from build123d import *

# Parameters (mm, degrees)
SKETCH1_W           = 59.055
SKETCH1_H           = 28.448
BOSS_EXTRUDE1_DEPTH = 46.482
SKETCH2_R           = 2.54
BOSS_EXTRUDE2_DEPTH = 3.81
FILLET1_R           = 2.54
CHAMFER1_SIZE       = 1.778


with BuildPart() as part:
    # Sketch1 → Boss-Extrude1 (new body)
    with BuildSketch(Plane(origin=(0, 0, 0), x_dir=(1, 0, 0), z_dir=(0, 1, 0))):
        with Locations((-2.344011553, -9.758904569)):
            Rectangle(SKETCH1_W, SKETCH1_H)
    extrude(amount=BOSS_EXTRUDE1_DEPTH)

    # Sketch2 → Boss-Extrude2 (add)
    with BuildSketch(Plane(origin=(0, 46.482, 0), x_dir=(1, 0, 0), z_dir=(0, 1, 0))):
        with Locations(Location((14.483488447, -9.758904569, 0), (0, 0, 90))):
            Circle(SKETCH2_R)
    extrude(amount=BOSS_EXTRUDE2_DEPTH)

    # Fillet1
    fillet1_edges = [part.edges().sort_by_distance(p)[0] for p in [
        (-31.871511553, 23.241, -4.465095431),
        (27.183488447, 23.241, -4.465095431),
        (27.183488447, 23.241, 23.982904569),
        (-31.871511553, 23.241, 23.982904569),
    ]]
    fillet(fillet1_edges, radius=FILLET1_R)

    # Chamfer1
    chamfer1_edges = [part.edges().sort_by_distance(p)[0] for p in [
        (-31.871511553, 0, 9.758904569),
        (-2.344011553, 0, -4.465095431),
        (27.183488447, 0, 9.758904569),
        (-2.344011553, 0, 23.982904569),
        (-31.127562777, 0, 23.238955793),
        (26.439539672, 0, 23.238955793),
        (26.439539672, 0, -3.721146655),
        (-31.127562777, 0, -3.721146655),
    ]]
    chamfer(chamfer1_edges, length=CHAMFER1_SIZE)


solid = part.part
Could you check a few things on this model? Use its own coordinates, in mm. Round coordinates to 2 decimals unless told otherwise and drop trailing zeros. Write each loop counter-clockwise with the first axis right and the second up, starting at its lowest first coordinate (ties: lowest second). Pieces come first, ordered by that corner, then holes. Notation, with made-up numbers: (89, 60.25) - (112, 60.25) arc R14 cw to (112, 85.25) - close; hole circle Ø11 at (88.5, 7). An arc over 180 degrees is marked (long way). Put each result on its own line as item: value. Start each with the question number.
(1) I need wall thicknesses on probe 1 along Y at (x, z) = (3, 15.5); probe 2 along X at (y, z) = (35, 23.25); probe 3 along X at (y, z) = (5, 22.75). Which ranges of each line are inside material? Lowest first, please.
(2) Thinking about a two-plate mould opening in X: for faces 1 (the flat face through (-2.722, 0.877, -3.564)), 2 (the flat face through (-30.97, 0.877, 9.922)), 3 (the cylindrical face through (14.372, 48.36, 12.296)), 4 (the cylindrical face through (26.42, 24.44, -3.74)), which applies, released by +X, released by -X, zero draft, split by the parting line, or undercut?
(3) Will this pin go through, and if not, where does the flat tip stop? pin 1 (14 mm diameter, centred on x = -4.5, z = 8.5, fed in from +Y).
(4) I want a section at D-D, the plane x = 13. Please give me the cut outline in (y, z).
(5) I want a section at A-A, the plane x = -13. Please give me the cut outline in (y, z).
(6) I want a section at C-C, the plane z = 9.75. Please give me the cut outline in (x, y).
(7) I want a section at B-B, the plane z = 20.25. Please give me the cut outline in (x, y), plus the area to 3 significant figures.
Here are the results:
1. probe 1: y = 0 to 46.48
1. probe 2: x = -31.12 to 26.43
1. probe 3: x = -31.51 to 26.82
2. face 1: zero draft
2. face 2: released by -X
2. face 3: split by the parting line
2. face 4: released by +X
3. pin 1: stops at y = 46.48
4. outline: (0, -2.69) - (1.78, -4.47) - (46.48, -4.47) - (46.48, 7.7) - (50.29, 7.7) - (50.29, 11.82) - (46.48, 11.82) - (46.48, 23.98) - (1.78, 23.98) - (0, 22.2) - close
5. outline: (0, -2.69) - (1.78, -4.47) - (46.48, -4.47) - (46.48, 23.98) - (1.78, 23.98) - (0, 22.2) - close
6. outline: (-31.87, 1.78) - (-30.09, 0) - (25.41, 0) - (27.18, 1.78) - (27.18, 46.48) - (17.02, 46.48) - (17.02, 50.29) - (11.94, 50.29) - (11.94, 46.48) - (-31.87, 46.48) - close
7. outline: (-31.87, 1.78) - (-30.09, 0) - (25.41, 0) - (27.18, 1.78) - (27.18, 46.48) - (-31.87, 46.48) - close
7. area: 2,740 mm^2
